Geometry: see drawing. Coordinates: mm, zero at the bounding-box minimum. A direction names the side the tool comes from. Coordinates: 2 decimals unless noted, no trailing zeros. Loops run counter-clockwise (first coordinate to the right, second up) from the corner with the lowest first, then second, coordinate; pieces in that order, holes last. Notation, with made-up numbers: (0, 14.25) - (59, 14.25) arc R18 ccw to (59, 46.25) - close; hole circle Ø7 at (-24.75, 0). An arc over 180 degrees is marked (long way). Use one line per item in the form item = value.
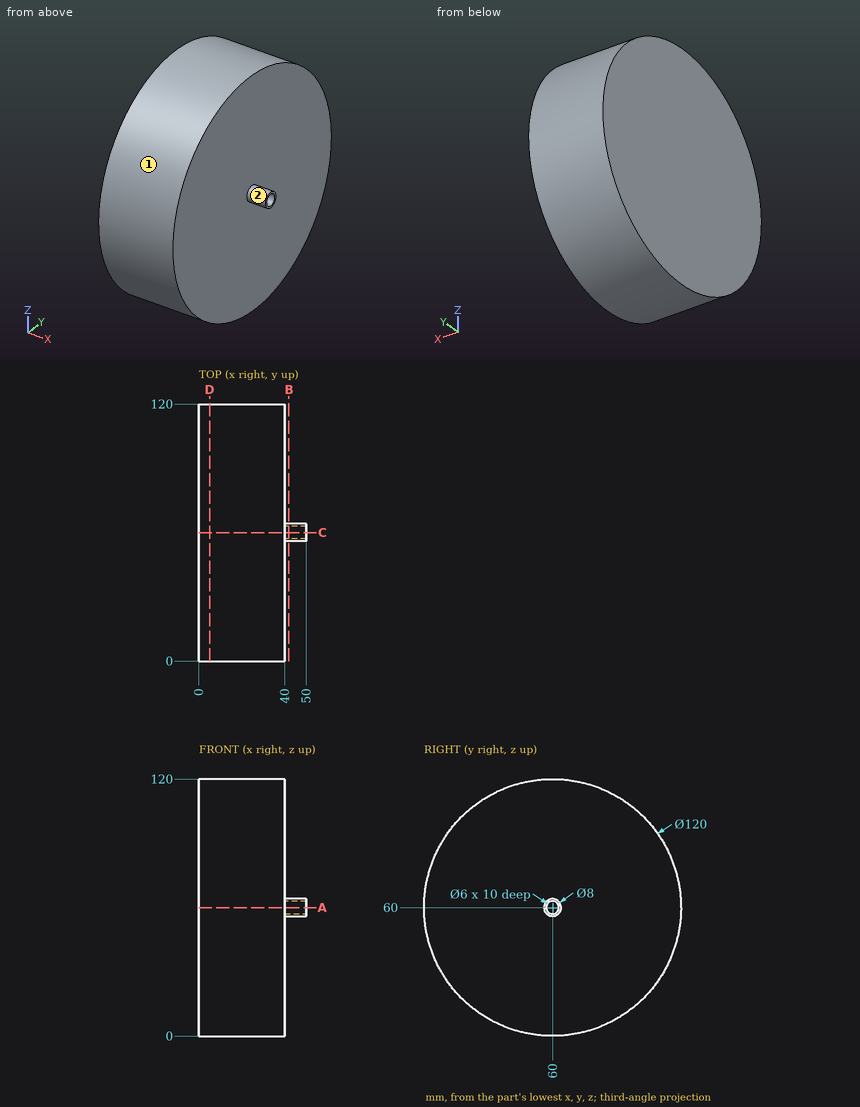
Q1. Set-up query: the marked faces 1 and 2. Return all of +Z, -Z, +X, -X, +Y, -Y with unobstructed straight access to the full face (end or side cutting, diameter ignored); none if empty.
Check values:
face_1 = +X, -X
face_2 = +X
Q2. Cut plane A-A, the plane z = 60. Return loops of the section in (x, y), then the cut area to 3 significant figures.
Check values:
outline = (0, 0) - (40, 0) - (40, 56) - (50, 56) - (50, 57) - (40, 57) - (40, 63) - (50, 63) - (50, 64) - (40, 64) - (40, 120) - (0, 120) - close
area = 4,820 mm²
Q3. First-contact query: P1, Ø10, axis at x = 12, z = 54.5, coming from the +Y side; P2, Ø5, axis at x = 36.5, z = 82, coming from the -Y side; P3, Ø1.8, axis at y = 61, z = 60.5, coming from the +X side. Flat tips, straight axial feed; report the tip coordinate or a pass-through.
Check values:
P1 = 120
P2 = 3.26
P3 = 40
Q4. Ray query, line 1 along Y through (x, z) = (42.5, 60); line 2 along X through (y, z) = (12, 70); line 3 along Z through (x, y) = (6, 61). Return the intervals inside material, ascending. Write a range as [from, to].
Check values:
line_1 = [56, 57], [63, 64]
line_2 = [0, 40]
line_3 = [0.01, 119.99]
Q5. Cut plane D-D, the plane x = 5. Return loops of the section in (y, z), then the cut area to 3 significant figures.
Check values:
outline = circle Ø120 at (60, 60)
area = 11,300 mm²
Q6. Cut plane B-B, the plane x = 42. Return loops of the section in (y, z).
Check values:
outline = circle Ø8 at (60, 60); hole circle Ø6 at (60, 60)
